Job drawing, mm, ordinate dimensions from the low corner. One solid piece. A direction names the side the tool comes from. Coordinates: 2 decimals unless noted, no trailing zeros. Order: outer loops, then holes, each group sorted by start corner. A loop starts at its lowest first (then second) coordinate and runs counter-clockwise, first axis right, second up. Notation, with made-up numbers: (-33.75, 75.25) -> (7.25, 75.25) arc R24 cw to (7.25, 103.25) -> close; hole circle Ø2 at (86, -14.75). An arc over 180 degrees is marked (long way). Use CSV: the item, a comma, the result in double quotes. Start each with the question number.
(1) Cut at A-A on z = 39. Write the cut outline in (x, y).
(2) Tool access for the marked faces 4, 5, 6, 7 and 8: list every direction of +Z, -Z, +X, -X, +Y, -Y with a clear straight run to the whole face (end or side of a thin tool).
(3) Cut at B-B on y = 11.5. Give the number of separate pieces and of enclosed holes in the cut face, plus the area to 3 significant figures.
(4) Cut at C-C on x = 20. Write the cut outline in (y, z).
(5) Probe L1, parallel to Y at x = 28.5, z = 39; L2, parallel to Z at x = 5, y = 22; L3, parallel to Y at x = 24, z = 40.5. List the from-to ranges inside material, lowest first.
(6) Pin check, flat tips, straight feed: pin 1 Ø10 at (x, z) = (26, 37) entering from +Y; pin 2 Ø22 at (x, z) = (25, 28.5) entering from -Y; pin 3 Ø4 at (x, y) = (18, 17) entering from -Z; pin 4 Ø2 at (y, z) = (20, 31.5) entering from +X. Stop position of each tip, or through.
(7) Pull direction X, two halves, no side cores. Call the marked faces 1, 2 and 3: pulls with the +X half, pulls with the -X half, needs draft (parallel to the pull), parting line crosses it, or undercut.
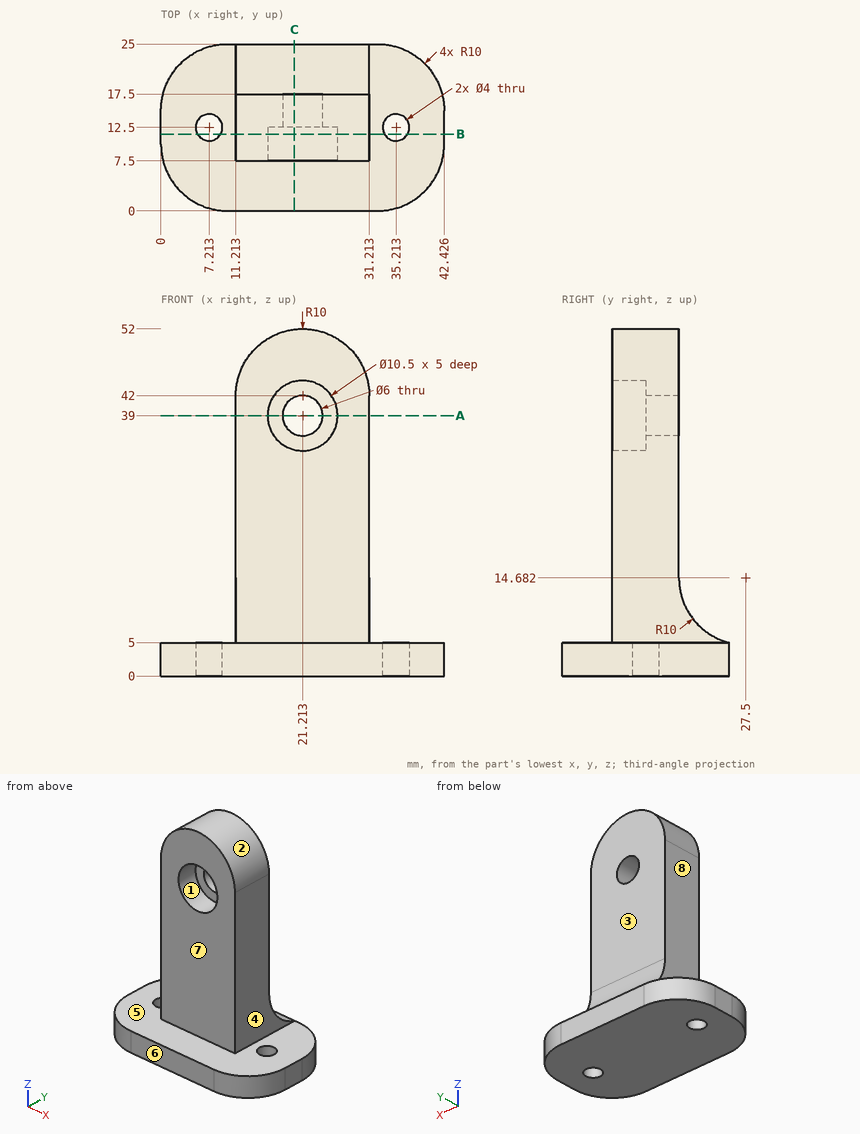
Outcome:
1,outline,"(11.21, 7.5) -> (15.96, 7.5) -> (15.96, 12.5) -> (18.21, 12.5) -> (18.21, 17.5) -> (11.21, 17.5) -> close; (24.21, 12.5) -> (26.46, 12.5) -> (26.46, 7.5) -> (31.21, 7.5) -> (31.21, 17.5) -> (24.21, 17.5) -> close"
2,face 4,"+Z, +X, +Y, -Y"
2,face 5,"+Z, -Y"
2,face 6,"+Z, -Z, +X, -X, -Y"
2,face 7,"+Z, +X, -X, -Y"
2,face 8,"+Z, -X, +Y, -Y"
3,separate pieces,"3"
3,enclosed holes,"1"
3,area,"988 mm2"
4,outline,"(0, 0) -> (25, 0) -> (25, 5) arc R10 cw to (17.5, 14.68) -> (17.5, 36.26) -> (12.5, 36.26) -> (12.5, 33.89) -> (7.5, 33.89) -> (7.5, 5) -> (0, 5) -> close; (7.5, 44.11) -> (12.5, 44.11) -> (12.5, 41.74) -> (17.5, 41.74) -> (17.5, 51.93) -> (7.5, 51.93) -> close"
5,L1,"7.5 to 17.5"
5,L2,"0 to 5"
5,L3,"12.5 to 17.5"
6,pin 1,"y = 17.5"
6,pin 2,"y = 7.5"
6,pin 3,"z = 0"
6,pin 4,"through"
7,face 1,"undercut"
7,face 2,"parting line crosses it"
7,face 3,"needs draft"
